Work out the finished part from the listing and answer in its coordinate system (mm). A direction names the side the tool comes from. Give positions to 0.01 mm unless a question says otherwise; leave off trailing zeros. Loops run counter-clockwise (first coordinate to the right, second up) from the corner with the lowest first, then second, coordinate; pieces in that order, holes last. Notation, with made-up numbers: (5, 35) -> (22, 35) arc R7 cw to (22, 44) -> close; hole circle Ø8 at (88.5, -30.5). An arc over 180 degrees is marked (long way). Answer as CSV lines item,"result". Start each with the question number.
1. Find section D-D, the plane y = -46. Give the vertices of the cut face in (x, z), and give its area (3 significant figures).
2. Find section A-A, the plane x = 0. Count the separate pieces of the cut face and the enclosed holes in it, and give its area (3 significant figures).
3. Flat-ended cylindrical pins translate along their axes: pin 1 Ø1 at (x, y) = (-2, 30.5) entering from +Z; pin 2 Ø2 at (x, z) = (-4, 3) entering from +Y; pin 3 Ø2 at (x, z) = (3, 1) entering from +Y. Find the tip coordinate at first contact, or state that the pin passes through.
4. Find the intervals of material crossed by line 1 along X through (y, z) = (35, 1); line 2 along X through (y, z) = (-17, 2.9); line 3 along Y through (x, z) = (0, 4.4), in increasing order.
5. Find section B-B, the plane y = 41. Give the vertices of the cut face in (x, z), and give its area (3 significant figures).
6. A tool of negligible diameter and unlimited length cuts with its end or side. For faces 1 (the face through (-1, -9, 2)), 2 (the face through (-0.46, 51.95, 4.49)), 3 (the face through (0, -64, 2)), from which of +Z, -Z, +X, -X, +Y, -Y can it reach the whole face along a straight path? Write none if from no direction.
7. Determine the mould class of faces 4 (the face through (-6, -19, 2)), 5 (the face through (0, 64, 2)), 6 (the face through (2, 56, 5)) for opening direction Y: +Y half, -Y half, draft (parallel to the pull), parting line (faces both ways), or undercut.
from build123d import *

# Parameters (mm, degrees)
CROQUIS1_R              = 2.1
SALIENTE_EXTRUIR1_DEPTH = 4
CROQUIS1_6_R            = 2.1
SALIENTE_EXTRUIR3_DEPTH = 5
REDONDEO1_R             = 1


with BuildPart() as part:
    # Croquis1 → Saliente-Extruir1 (new body)
    with BuildSketch(Plane.XY):
        with BuildLine():
            ThreePointArc((10, 54), (0, 64), (-10, 54))
            Line((-10, 54), (-10, -54))
            ThreePointArc((-10, -54), (0, -64), (10, -54))
            Line((10, -54), (10, 54))
        make_face()
        with BuildLine():
            Line((6, 38), (6, 22))
            Line((6, 22), (-6, 34))
            Line((-6, 34), (-6, 38))
            ThreePointArc((-6, 38), (0, 44), (6, 38))
        make_face(mode=Mode.SUBTRACT)
        Polygon((6, 16), (6, -16), (-6, -4), (-6, 4), align=None, mode=Mode.SUBTRACT)
        with BuildLine():
            Line((6, -22), (6, -38))
            ThreePointArc((6, -38), (0, -44), (-6, -38))
            Line((-6, -38), (-6, -34))
            Line((-6, -34), (6, -22))
        make_face(mode=Mode.SUBTRACT)
        Polygon((-6, -31), (-6, -7), (6, -19), align=None, mode=Mode.SUBTRACT)
        Polygon((-6, 7), (-6, 31), (6, 19), align=None, mode=Mode.SUBTRACT)
        with Locations((0, -54)):
            Circle(CROQUIS1_R, mode=Mode.SUBTRACT)
    extrude(amount=SALIENTE_EXTRUIR1_DEPTH)

    # Croquis1_6 → Saliente-Extruir3 (add)
    with BuildSketch(Plane.XY):
        with BuildLine():
            Line((10, 47.95), (10, 54))
            ThreePointArc((10, 54), (0, 64), (-10, 54))
            Line((-10, 54), (-10, 47.95))
            Line((-10, 47.95), (10, 47.95))
        make_face()
        with Locations((0, 54)):
            Circle(CROQUIS1_6_R, mode=Mode.SUBTRACT)
    extrude(amount=SALIENTE_EXTRUIR3_DEPTH)

    # Redondeo1
    redondeo1_edges = [part.edges().sort_by_distance(p)[0] for p in [
        (6, 22, 2),
        (-6, 34, 2),
        (6, -22, 2),
        (-6, -34, 2),
        (-6, -31, 2),
        (6, -19, 2),
        (-6, -7, 2),
        (-6, -4, 2),
        (6, -16, 2),
        (6, 16, 2),
        (-6, 4, 2),
        (-6, 7, 2),
        (6, 19, 2),
        (-6, 31, 2),
    ]]
    fillet(redondeo1_edges, radius=REDONDEO1_R)


solid = part.part
Resolved:
1,outline,"(-10, 0) -> (10, 0) -> (10, 4) -> (-10, 4) -> close"
1,area,"80.0 mm^2"
2,separate pieces,"7"
2,enclosed holes,"0"
2,area,"203 mm^2"
3,pin 1,"stops at z = 4"
3,pin 2,"stops at y = 63.54"
3,pin 3,"stops at y = 63.8"
4,line 1,"x = -10 to -6, 6 to 10"
4,line 2,"x = -10 to -6, 4 to 10"
4,line 3,"y = 47.95 to 51.9, 56.1 to 64"
5,outline,"(-10, 0) -> (-5.2, 0) -> (-5.2, 4) -> (-10, 4) -> close; (5.2, 0) -> (10, 0) -> (10, 4) -> (5.2, 4) -> close"
5,area,"38.4 mm^2"
6,face 1,"+Z, -Z"
6,face 2,"+Z"
6,face 3,"+Z, -Z, -Y"
7,face 4,"undercut"
7,face 5,"+Y half"
7,face 6,"draft"
